from build123d import *

# Parameters (mm, degrees)
BOSS_EXTRUDE1_DEPTH = 27.5
CUT_EXTRUDE1_DEPTH  = 55
SKETCH3_R           = 10.5
CUT_EXTRUDE2_DEPTH  = 85
SKETCH4_R           = 16
SKETCH4_R_2         = 10.5
CUT_EXTRUDE3_DEPTH  = 32.3
CUT_EXTRUDE4_START  = -32.3
SKETCH5_R           = 16
SKETCH5_R_2         = 10.5
CUT_EXTRUDE4_DEPTH  = 32.3
SKETCH6_R           = 2.75
CUT_EXTRUDE5_DEPTH  = 15
SKETCH9_R           = 3.5
CUT_EXTRUDE6_DEPTH  = 15


with BuildPart() as part:
    # Sketch1 → Boss-Extrude1 (new, symmetric)
    with BuildSketch(Plane.XY):
        Polygon((0, 0), (0, -49), (-14.142135624, -63.142135624), (-70.857864376, -63.142135624), (-85, -49), (-85, 0), align=None)
    extrude(amount=BOSS_EXTRUDE1_DEPTH, both=True)

    # Sketch2 → Cut-Extrude1 (cut)
    with BuildSketch(Plane.XY.offset(27.5)):
        with BuildLine():
            Line((-36.843145751, 0), (-48.156854249, 0))
            ThreePointArc((-48.156854249, 0), (-42.5, -8), (-36.843145751, 0))
        make_face()
    extrude(amount=-CUT_EXTRUDE1_DEPTH, mode=Mode.SUBTRACT)

    # Sketch3 → Cut-Extrude2 (cut)
    with BuildSketch(Plane(origin=(0, 0, 0), x_dir=(0, 0, -1), z_dir=(1, 0, 0))):
        with Locations(Location((0, -24.5, 0), (0, 0, 90))):
            Circle(SKETCH3_R)
    extrude(amount=-CUT_EXTRUDE2_DEPTH, mode=Mode.SUBTRACT)

    # Sketch4 → Cut-Extrude3 (cut)
    with BuildSketch(Plane(origin=(0, 0, 0), x_dir=(0, 0, -1), z_dir=(1, 0, 0))):
        with Locations(Location((0, -24.5, 0), (0, 0, 90))):
            Circle(SKETCH4_R)
        with Locations(Location((0, -24.5, 0), (0, 0, 90))):
            Circle(SKETCH4_R_2, mode=Mode.SUBTRACT)
    extrude(amount=-CUT_EXTRUDE3_DEPTH, mode=Mode.SUBTRACT)

    # Sketch5 → Cut-Extrude4 (cut)
    with BuildSketch(Plane.ZY.offset(85).offset(CUT_EXTRUDE4_START)):
        with Locations(Location((0, -24.5, 0), (0, 0, 90))):
            Circle(SKETCH5_R)
        with Locations(Location((0, -24.5, 0), (0, 0, 90))):
            Circle(SKETCH5_R_2, mode=Mode.SUBTRACT)
    extrude(amount=CUT_EXTRUDE4_DEPTH, mode=Mode.SUBTRACT)

    # Sketch6 → Cut-Extrude5 (cut)
    with BuildSketch(Plane(origin=(0, 0, 0), x_dir=(1, 0, 0), z_dir=(0, 1, 0))):
        with Locations(Location((-8, 19.5, 0), (0, 0, 180))):
            Circle(SKETCH6_R)
        with Locations((-8, -19.5)):
            Circle(SKETCH6_R)
        with Locations(Location((-77, -19.5, 0), (0, 0, 180))):
            Circle(SKETCH6_R)
        with Locations((-77, 19.5)):
            Circle(SKETCH6_R)
    extrude(amount=-CUT_EXTRUDE5_DEPTH, mode=Mode.SUBTRACT)

    # Loft1: read off the stored shape, not the designer's step
    # Loft1: loft between two sections, ruled curve by curve
    loft1_from = [
        Edge.make_bspline([(-20.976227121, -31.727080746, 27.5), (-43.806336876, -21.539534988, 27.5), (-53.993882634, -44.369644744, 27.5), (-31.163772879, -54.557190501, 27.5), (-8.333663124, -64.744736259, 27.5), (1.853882634, -41.914626504, 27.5), (-20.976227121, -31.727080746, 27.5)], [0, 0, 0, 0, 0.5, 0.5, 0.5, 1, 1, 1, 1], 3, [1, 0.333333333, 0.333333333, 1, 0.333333333, 0.333333333, 1]),
    ]
    loft1_to = [
        Edge.make_bspline([(-20.63774875, -37.26926185, 32.35), (-32.383496297, -26.40475935, 32.35), (-43.247998797, -38.150506897, 32.35), (-31.50225125, -49.015009397, 32.35), (-19.756503703, -59.879511897, 32.35), (-8.892001203, -48.13376435, 32.35), (-20.63774875, -37.26926185, 32.35)], [0, 0, 0, 0, 0.5, 0.5, 0.5, 1, 1, 1, 1], 3, [1, 0.333333333, 0.333333333, 1, 0.333333333, 0.333333333, 1]),
    ]
    loft1 = Solid(Shell([*[Face.make_surface_from_curves(loft1_from[k], loft1_to[k]) for k in range(1)], Face(Wire(loft1_from)), Face(Wire(loft1_to))]))
    add(loft1)

    # Sketch9 → Cut-Extrude6 (cut)
    with BuildSketch(Plane.XY.offset(32.35)):
        with Locations((-26.07, -43.142135624)):
            Circle(SKETCH9_R)
    cut_extrude6 = extrude(amount=-CUT_EXTRUDE6_DEPTH, mode=Mode.SUBTRACT)

    # Mirror1: Loft1, Cut-Extrude6 across plane
    add(loft1.mirror(Plane(origin=(-42.5, 0, 0), x_dir=(0, 0, 1), z_dir=(1, 0, 0))))
    add(cut_extrude6.mirror(Plane(origin=(-42.5, 0, 0), x_dir=(0, 0, 1), z_dir=(1, 0, 0))), mode=Mode.SUBTRACT)


solid = part.part
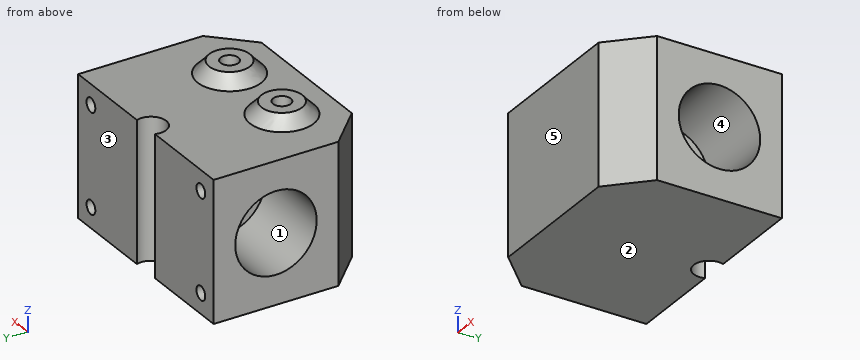
Source: CAD feature listing. Evaluate the final solid. Frame: model axes, mm. Face numbers are marked on the shaded views. A direction names the side the tool comes from. Round coordinates to 2 decimals unless told otherwise and drop trailing zeros. Loops run counter-clockwise (first coordinate to the right, second up) from the corner with the lowest first, then second, coordinate; pieces in that order, holes last. Notation, with made-up numbers: (23, -8.75) -> (28, -8.75) arc R13 cw to (28, 2.25) -> close; hole circle Ø4 at (-22.5, 9.25). An arc over 180 degrees is marked (long way). Answer as a JSON object with one key per item and string values. Group by question number.
Q1. Mould query, pull axis Z, two halves, no side actions, for the marked faces 1, 2 and 3. Classes: pulls with the +Z half, pulls with the -Z half, needs draft (parallel to the pull), parting line crosses it, or undercut.
Q2. Section query C-C (y = -24.5). Output: boundary loops of the cut face in (x, z).
Q3. Section query D-D (x = -77). Output: boundary loops of the cut face in (y, z), plus the area to 3 significant figures.
Q4. Ray query, line 1 (X direction, y = -9, z = 19); line 2 (Z direction, x = -77, y = -12); line 3 (Z direction, x = -81, y = -4). Return the intervals inside material, ascending. Write a range as from..to.
Q5. Section query A-A (y = -2). Output: boundary loops of the cut face in (x, z).
Q6. Contact query for flat-ended pins moving along their axis: P1, Ø3.5, axis at x = -77, z = -19.5, coming from the -Y side; P2, Ø1.6, axis at x = -76, z = -18.5, coming from the +Y side; P3, Ø5, axis at x = -66.5, y = -27, coming from the +Z side; P4, Ø12.5, axis at y = -24.5, z = 0, coming from the +X side. Output: stop coordinate, or through.
Q7. Access query for the marked faces 4 and 5. Directions: +Z, -Z, +X, -X, +Y, -Y. A direction counts if a zero-diameter tool reaches every point of the face in a straight line with its end or side. Return the directions, or none.
Q8. Section query B-B (z = 0). Output: boundary loops of the cut face in (x, y), plus the area to 3 significant figures.
Completed:
{
 "1": {"face 1": "undercut", "face 2": "pulls with the -Z half", "face 3": "needs draft"},
 "2": {"outline": "(-85, -27.5) -> (0, -27.5) -> (0, -16) -> (-32.3, -16) -> (-32.3, -10.5) -> (-52.7, -10.5) -> (-52.7, -16) -> (-85, -16) -> close; (-85, 16) -> (-52.7, 16) -> (-52.7, 10.5) -> (-32.3, 10.5) -> (-32.3, 16) -> (0, 16) -> (0, 27.5) -> (-85, 27.5) -> close"},
 "3": {"outline": "(-57, -27.5) -> (0, -27.5) -> (0, -22.25) -> (-15, -22.25) -> (-15, -16.75) -> (0, -16.75) -> (0, 16.75) -> (-15, 16.75) -> (-15, 22.25) -> (0, 22.25) -> (0, 27.5) -> (-57, 27.5) -> close; hole circle Ø32 at (-24.5, 0)", "area": "2,170 mm²"},
 "4": {"line 1": "-85..-79.7, -74.3..-10.7, -5.3..0", "line 2": "-27.5..-22.25, -16.75..-9.99, 9.99..16.75, 22.25..27.5", "line 3": "-27.5..27.5"},
 "5": {"outline": "(-85, -27.5) -> (-48.5, -27.5) -> (-48.5, 27.5) -> (-85, 27.5) -> close; (-36.5, -27.5) -> (0, -27.5) -> (0, 27.5) -> (-36.5, 27.5) -> close; hole circle Ø5.5 at (-77, -19.5); hole circle Ø5.5 at (-77, 19.5); hole circle Ø5.5 at (-8, -19.5); hole circle Ø5.5 at (-8, 19.5)"},
 "6": {"P1": "y = -58.75", "P2": "y = -15", "P3": "z = 27.5", "P4": "through"},
 "7": {"face 4": "+X", "face 5": "+Z, -Z, +X, -X, -Y"},
 "8": {"outline": "(-85, -49) -> (-70.86, -63.14) -> (-14.14, -63.14) -> (0, -49) -> (0, -40.5) -> (-32.3, -40.5) -> (-32.3, -35) -> (-52.7, -35) -> (-52.7, -40.5) -> (-85, -40.5) -> close; (-85, -8.5) -> (-52.7, -8.5) -> (-52.7, -14) -> (-32.3, -14) -> (-32.3, -8.5) -> (0, -8.5) -> (0, 0) -> (-36.84, 0) arc R6 cw (long way) to (-48.16, 0) -> (-85, 0) -> close", "area": "2,590 mm²"}
}
